Check sheet for the modelled part. Datum: model origin and axes. Units: mm. Face numbers are marked on the shaded views. Coordinates: 2 decimals unless noted, no trailing zeros. Order: outer loops, then holes, each group sorted by start corner. A loop starts at its lowest first (then second) coordinate and runs counter-clockwise, first axis right, second up.
from build123d import *

# Parameters (mm, degrees)
F0_W     = 177.8
F0_H     = 177.8
F0_R     = 38.1
F1_DEPTH = 25.4
F2_SIZE  = 25.4


with BuildPart() as f1:
    # F0 (on Front) → F1 (new body)
    with BuildSketch(Plane.XZ):
        with Locations((2.04625, 4.972448)):
            Rectangle(F0_W, F0_H)
        Circle(F0_R, mode=Mode.SUBTRACT)
    extrude(amount=F1_DEPTH)

    # F2
    f2_edges = [f1.edges().sort_by_distance(p)[0] for p in [
        (90.94625, -12.7, 93.872448),
    ]]
    chamfer(f2_edges, length=F2_SIZE)


solid = f1.part
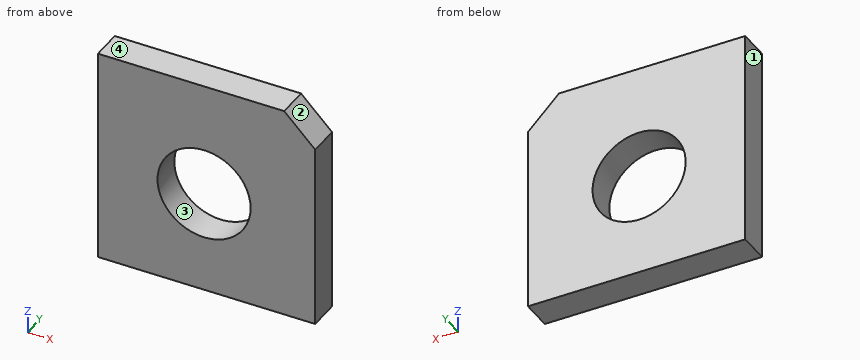
(1) Thickness scan on probe 1 along Z at (x, y) = (0, -17.5); probe 2 along Z at (x, y) = (-10, -4.25); probe 3 along X at (y, z) = (-12, 17). Record the ranges inside material, lowest first.
Filled in:
probe 1: z = -83.93 to -38.1, 38.1 to 93.87
probe 2: z = -83.93 to -36.76, 36.76 to 93.87
probe 3: x = -86.85 to -34.1, 34.1 to 90.95
(2) Cross-section at A-A (x = 0). Enter the section's corners in (y, z).
Filled in:
outline: (-25.4, -83.93) - (0, -83.93) - (0, -38.1) - (-25.4, -38.1) - close; (-25.4, 38.1) - (0, 38.1) - (0, 93.87) - (-25.4, 93.87) - close
(3) Cross-section at C-C (y = -21). Enter the section's corners in (x, z).
Filled in:
outline: (-86.85, -83.93) - (90.95, -83.93) - (90.95, 68.47) - (65.55, 93.87) - (-86.85, 93.87) - close; hole circle Ø76.2 at (0, 0)
(4) Cross-section at B-B (z = 0). Enter the section's corners in (x, y).
Filled in:
outline: (-86.85, -25.4) - (-38.1, -25.4) - (-38.1, 0) - (-86.85, 0) - close; (38.1, -25.4) - (90.95, -25.4) - (90.95, 0) - (38.1, 0) - close
(5) Release check for a two-part mould opening along X. For the marked faces 1, 2, 3 and 4 record: +X half, -X half, draft (parallel to the pull), parting line (faces both ways), or undercut.
Filled in:
face 1: -X half
face 2: +X half
face 3: undercut
face 4: draft
(6) Go/stop test with a flat-tipped pin: P1, Ø5, axis at x = -65.5, z = -11, coming from the +Y side. Record where the tip stops, or that it passes through.
Filled in:
P1: stops at y = 0
(7) Cross-section at D-D (x = 71). Enter the section's corners in (y, z), and give its area (3 significant figures).
Filled in:
outline: (-25.4, -83.93) - (0, -83.93) - (0, 88.42) - (-25.4, 88.42) - close
area: 4,380 mm2
